Part model, mm, in its own coordinate system. A direction names the side the tool comes from. Coordinates: 2 decimals unless noted, no trailing zeros. Loops run counter-clockwise (first coordinate to the right, second up) from the corner with the lowest first, then second, coordinate; pieces in that order, holes last. Notation, with made-up numbers: M -24.75,47.5 L -6.75,47.5 A24 cw -6.75,72.5 Z; hole C 60,9.25 d7. An arc over 180 degrees is marked long. Use CSV: the item, a comma, the result in double quotes. Start each with the question number.
Autodesk Inventor part; units mm, degrees
ref_plane "YZ Plane" through (0, 0, 0) normal (1, 0, 0) x (0, 1, 0)
ref_plane "XZ Plane" through (0, 0, 0) normal (0, 1, 0) x (-1, 0, 0)
ref_plane "XY Plane" through (0, 0, 0) normal (0, 0, 1) x (1, 0, 0)
sketch "Skizze1" plane through (0, 0, 0) normal (0, 0, 1) x (1, 0, 0)
  circle A0 centre (0, 0) radius 15.5
  dimension "d0" = 31
extrude "Extrusion1" add sketch "Skizze1" along normal blind 11
sketch "Skizze2" plane through (0, 0, 11) normal (0, 0, 1) x (1, 0, 0)
  line L0 (-2.5, -2.5) -> (2.5, -2.5)
  line L1 (2.5, -2.5) -> (2.5, 2.5)
  line L2 (2.5, 2.5) -> (-2.5, 2.5)
  line L3 (-2.5, 2.5) -> (-2.5, -2.5)
  line L4 (-2.5, -2.5) -> (2.5, 2.5) construction
  line L5 (2.5, -2.5) -> (-2.5, 2.5) construction
  circle A0 centre (0, 0) radius 3
  dimension "d3" = 5
  dimension "d14" = 6
extrude "Extrusion2" cut sketch "Skizze2" against normal blind 2.5 contours A0 L3 L2 L1 L0 | L0 A0 | A0 L3 | L1 A0 | A0 L2
sketch "Skizze3" plane through (0, 0, 11) normal (0, 0, 1) x (1, 0, 0)
  circle A0 centre (0, 0) radius 11.25
  line L0 (-7.955, -7.955) -> (7.955, -7.955)
  line L1 (7.955, -7.955) -> (7.955, 7.955)
  line L2 (7.955, 7.955) -> (-7.955, 7.955)
  line L3 (-7.955, 7.955) -> (-7.955, -7.955)
  line L4 (-7.955, -7.955) -> (7.955, 7.955) construction
  line L5 (7.955, -7.955) -> (-7.955, 7.955) construction
  dimension "d6" = 22.5
hole "Bohrung1" at (-7.955, -7.955, 11) at (7.955, -7.955, 11) at (7.955, 7.955, 11) at (-7.955, 7.955, 11) direction (0, 0, -1) diameter 3 end through all counterbore diameter 6 counterbore depth 5
properties part number "rotBaseMagnetMount" material "ABS-Kunststoff"
1. Tool access for faces 1 (the face through (-5.026, -7.305, 8.465)), 2 (the face through (-7.38, -9.34, 2.96)): list every direction of +Z, -Z, +X, -X, +Y, -Y with a clear straight run to the whole face (end or side of a thin tool).
2. Slice it at D-D, the plane x = 7.5. List the corners of the cut face in (y, z), and give its area (3 significant figures).
3. Pin check, flat tips, straight feed: pin 1 (1.8 mm diameter, centred on x = 1, y = -1.5, fed in from +Z); pin 2 (2 mm diameter, centred on y = -6, z = 5.5, fed in from -X); pin 3 (5 mm diameter, centred on x = -4.5, z = 6.5, fed in from -Y). Stop position of each tip, or through.
4. Wall check: probe 1 along X at (y, z) = (10.5, 9.25); probe 2 along Y at (x, z) = (-7.5, 8); probe 3 along Y at (x, z) = (6, 9). Give the ranges that are in metal, low to high.
5. Slice it at C-C, the plane y = 8. List the corners of the cut face in (x, z), and give its area (3 significant figures).
6. Two-plate mould, pull along Y, no slides. Class faces 3 (the face through (0, 0, 0)), 4 (the face through (-2.018, -15.368, 5.423)), 5 (the face through (9.2, 6.7, 6)): pulls with the +Y half, pulls with the -Y half, needs draft (parallel to the pull), parting line crosses it, or undercut.
7. Slice it at A-A, the plane y = 0. List the corners of the cut face in (x, z).
Found:
1,face 1,"+Z"
1,face 2,"+Z, -Z"
2,outline,"M -13.56,0 L -9.38,0 L -9.38,6 L -10.92,6 L -10.92,11 L -13.56,11 Z; M -6.53,0 L 6.53,0 L 6.53,6 L 4.99,6 L 4.99,11 L -4.99,11 L -4.99,6 L -6.53,6 Z; M 9.38,0 L 13.56,0 L 13.56,11 L 10.92,11 L 10.92,6 L 9.38,6 Z"
2,area,"205 mm^2"
3,pin 1,"z = 8.5"
3,pin 2,"x = -14.67"
3,pin 3,"y = -15.37"
4,probe 1,"-11.4 to -9.54, -6.37 to 6.37, 9.54 to 11.4"
4,probe 2,"-13.56 to -10.92, -4.99 to 4.99, 10.92 to 13.56"
4,probe 3,"-14.29 to -10.23, -5.68 to 5.68, 10.23 to 14.29"
5,outline,"M -13.28,0 L -9.45,0 L -9.45,6 L -10.95,6 L -10.95,11 L -13.28,11 Z; M -6.46,0 L 6.46,0 L 6.46,6 L 4.96,6 L 4.96,11 L -4.96,11 L -4.96,6 L -6.46,6 Z; M 9.45,0 L 13.28,0 L 13.28,11 L 10.95,11 L 10.95,6 L 9.45,6 Z"
5,area,"196 mm^2"
6,face 3,"needs draft"
6,face 4,"parting line crosses it"
6,face 5,"undercut"
7,outline,"M -15.5,0 L 15.5,0 L 15.5,11 L 3,11 L 3,8.5 L -3,8.5 L -3,11 L -15.5,11 Z"
